```python
from build123d import *

# Parameters (mm, degrees)
BOSS_EXTRUDE1_DEPTH = 60
CUT_EXTRUDE1_DEPTH  = 10
CUT_EXTRUDE2_DEPTH  = 10
CUT_EXTRUDE3_DEPTH  = 30
SKETCH7_R           = 10
CUT_EXTRUDE5_DEPTH  = 75
SKETCH8_R           = 10
CUT_EXTRUDE6_DEPTH  = 75
SKETCH9_W           = 42
SKETCH9_H           = 40
CUT_EXTRUDE8_DEPTH  = 65
CUT_EXTRUDE9_DEPTH  = 10
CUT_EXTRUDE10_DEPTH = 20
SKETCH12_W          = 40
SKETCH12_H          = 10
CUT_EXTRUDE11_DEPTH = 20
BOSS_EXTRUDE2_DEPTH = 20
SKETCH14_R          = 10
CUT_EXTRUDE14_DEPTH = 20
CUT_EXTRUDE15_DEPTH = 10
BOSS_EXTRUDE3_DEPTH = 20
SKETCH18_R          = 10
CUT_EXTRUDE16_DEPTH = 20
CUT_EXTRUDE17_DEPTH = 10


with BuildPart() as part:
    # Sketch2 → Boss-Extrude1 (new body)
    with BuildSketch(Plane.XY):
        with BuildLine():
            Line((0, 0), (150, 0))
            Line((150, 0), (150, 70))
            Line((150, 70), (120, 70))
            Line((120, 70), (120, 40))
            Line((120, 40), (40, 40))
            ThreePointArc((40, 40), (11.715728753, 28.284271247), (0, 0))
        make_face()
    extrude(amount=BOSS_EXTRUDE1_DEPTH)

    # Sketch4 → Cut-Extrude1 (cut)
    with BuildSketch(Plane(origin=(150, 0, 0), x_dir=(0, 0, -1), z_dir=(1, 0, 0))):
        with BuildLine():
            Line((-50, 70), (-40, 70))
            ThreePointArc((-40, 70), (-30, 60), (-20, 70))
            Line((-20, 70), (-10, 70))
            ThreePointArc((-10, 70), (-30, 50), (-50, 70))
        make_face()
    extrude(amount=-CUT_EXTRUDE1_DEPTH, mode=Mode.SUBTRACT)

    # Sketch5 → Cut-Extrude2 (cut)
    with BuildSketch(Plane.ZY.offset(-120)):
        with BuildLine():
            Line((10, 70), (20, 70))
            ThreePointArc((20, 70), (30, 60), (40, 70))
            Line((40, 70), (50, 70))
            ThreePointArc((50, 70), (30, 50), (10, 70))
        make_face()
    extrude(amount=-CUT_EXTRUDE2_DEPTH, mode=Mode.SUBTRACT)

    # Sketch6 → Cut-Extrude3 (cut)
    with BuildSketch(Plane.ZY.offset(-120)):
        with BuildLine():
            Line((20, 70), (40, 70))
            ThreePointArc((40, 70), (30, 60), (20, 70))
        make_face()
    extrude(amount=-CUT_EXTRUDE3_DEPTH, mode=Mode.SUBTRACT)

    # Sketch7 → Cut-Extrude5 (cut)
    with BuildSketch(Plane(origin=(0, 40, 0), x_dir=(1, 0, 0), z_dir=(0, 1, 0))):
        with Locations((90, -30)):
            Circle(SKETCH7_R)
    extrude(amount=-CUT_EXTRUDE5_DEPTH, mode=Mode.SUBTRACT)

    # Sketch8 → Cut-Extrude6 (cut)
    with BuildSketch(Plane.XZ):
        with Locations((30, 30)):
            Circle(SKETCH8_R)
    extrude(amount=-CUT_EXTRUDE6_DEPTH, mode=Mode.SUBTRACT)

    # Sketch9 → Cut-Extrude8 (cut)
    with BuildSketch(Plane(origin=(0, 20, 0), x_dir=(1, 0, 0), z_dir=(0, 1, 0))):
        with Locations((29, -30)):
            Rectangle(SKETCH9_W, SKETCH9_H)
    extrude(amount=CUT_EXTRUDE8_DEPTH, mode=Mode.SUBTRACT)

    # Sketch10 → Cut-Extrude9 (cut)
    with BuildSketch(Plane(origin=(0, 40, 0), x_dir=(1, 0, 0), z_dir=(0, 1, 0))):
        with BuildLine():
            Line((90, -20), (50, -20))
            Line((50, -20), (50, -40))
            Line((50, -40), (90, -40))
            ThreePointArc((90, -40), (80, -30), (90, -20))
        make_face()
    extrude(amount=-CUT_EXTRUDE9_DEPTH, mode=Mode.SUBTRACT)

    # Sketch11 → Cut-Extrude10 (cut)
    with BuildSketch(Plane.XY.offset(20)):
        Polygon((50, 20), (70, 30), (50, 30), align=None)
    extrude(amount=CUT_EXTRUDE10_DEPTH, mode=Mode.SUBTRACT)

    # Sketch12 → Cut-Extrude11 (cut)
    with BuildSketch(Plane(origin=(0, 40, 0), x_dir=(1, 0, 0), z_dir=(0, 1, 0))):
        with Locations((90, -55)):
            Rectangle(SKETCH12_W, SKETCH12_H)
        with Locations((90, -5)):
            Rectangle(SKETCH12_W, SKETCH12_H)
    extrude(amount=-CUT_EXTRUDE11_DEPTH, mode=Mode.SUBTRACT)

    # Sketch13 → Boss-Extrude2 (add)
    with BuildSketch(Plane(origin=(0, 0, 0), x_dir=(1, 0, 0), z_dir=(0, 1, 0))):
        with BuildLine():
            Line((70, -70), (70, -80))
            ThreePointArc((70, -80), (90, -100), (110, -80))
            Line((110, -80), (110, -70))
            ThreePointArc((110, -70), (112.928932188, -62.928932188), (120, -60))
            Line((120, -60), (60, -60))
            ThreePointArc((60, -60), (67.071067812, -62.928932188), (70, -70))
        make_face()
    extrude(amount=BOSS_EXTRUDE2_DEPTH)

    # Sketch14 → Cut-Extrude14 (cut)
    with BuildSketch(Plane(origin=(0, 20, 0), x_dir=(1, 0, 0), z_dir=(0, 1, 0))):
        with Locations((90, -80)):
            Circle(SKETCH14_R)
    extrude(amount=-CUT_EXTRUDE14_DEPTH, mode=Mode.SUBTRACT)

    # Sketch15 → Cut-Extrude15 (cut)
    with BuildSketch(Plane(origin=(0, 20, 0), x_dir=(1, 0, 0), z_dir=(0, 1, 0))):
        with BuildLine():
            Line((70, -80), (80, -80))
            ThreePointArc((80, -80), (90, -90), (100, -80))
            Line((100, -80), (110, -80))
            ThreePointArc((110, -80), (90, -100), (70, -80))
        make_face()
    extrude(amount=-CUT_EXTRUDE15_DEPTH, mode=Mode.SUBTRACT)

    # Sketch17 → Boss-Extrude3 (add)
    with BuildSketch(Plane.XZ):
        with BuildLine():
            Line((110, -10), (110, -20))
            ThreePointArc((110, -20), (90, -40), (70, -20))
            Line((70, -20), (70, -10))
            ThreePointArc((70, -10), (67.071067812, -2.928932188), (60, 0))
            Line((60, 0), (120, 0))
            ThreePointArc((120, 0), (112.928932188, -2.928932188), (110, -10))
        make_face()
    extrude(amount=-BOSS_EXTRUDE3_DEPTH)

    # Sketch18 → Cut-Extrude16 (cut)
    with BuildSketch(Plane(origin=(0, 20, 0), x_dir=(1, 0, 0), z_dir=(0, 1, 0))):
        with Locations((90, 20)):
            Circle(SKETCH18_R)
    extrude(amount=-CUT_EXTRUDE16_DEPTH, mode=Mode.SUBTRACT)

    # Sketch19 → Cut-Extrude17 (cut)
    with BuildSketch(Plane(origin=(0, 20, 0), x_dir=(1, 0, 0), z_dir=(0, 1, 0))):
        with BuildLine():
            Line((100, 20), (110, 20))
            ThreePointArc((110, 20), (90, 40), (70, 20))
            Line((70, 20), (80, 20))
            ThreePointArc((80, 20), (90, 30), (100, 20))
        make_face()
    extrude(amount=-CUT_EXTRUDE17_DEPTH, mode=Mode.SUBTRACT)


solid = part.part
```
Source: CAD feature listing. Evaluate the final solid. Frame: model axes, mm. A direction names the side the tool comes from. Coordinates: 2 decimals unless noted, no trailing zeros. Loops run counter-clockwise (first coordinate to the right, second up) from the corner with the lowest first, then second, coordinate; pieces in that order, holes last. Notation, with made-up numbers: M 31,-12.5 L 71,-12.5 A5 ccw 71,-3.5 Z; hole C 59.25,81 d6. An arc over 180 degrees is marked long. Use a Markdown table: item, result. Add a question column.
Q1. Material intervals for L1, parallel to Z at x = 90, y = 9; L2, parallel to Z at x = 49, y = 36; L3, parallel to Z at x = 98, y = 6, sorted ascending.
Q2. Section query C-C, the plane y = 38. Return loops of the section in (x, z).
Q3. First-contact query: pin 1 (5 mm diameter, centred on x = 48, y = 13.5, fed in from +Z); pin 2 (12 mm diameter, centred on x = 30, z = 30, fed in from -Y); pin 3 (15 mm diameter, centred on y = 52.5, z = 28.5, fed in from -X); pin 4 (8 mm diameter, centred on x = 133, y = 18, fed in from -Z). Flat tips, straight axial feed; report the tip coordinate or a pass-through.
Q4. Section query D-D, the plane x = 30. Return loops of the section in (y, z).
Q5. Section query A-A, the plane z = 30. Return loops of the section in (x, y).
Q6. Section query B-B, the plane x = 82. Return loops of the section in (y, z).
Q7. Draft query along Z for faces 4 (the flat face through (50, 30, 15)), 5 (the cylindrical face through (90, 5, -40)), 6 (the flat face through (70, 10, -15)). Return one class per face: pulls with the +Z half, pulls with the -Z half, needs draft (parallel to the pull), parting line crosses it, or undercut.
Q8. Access query for faces 1 (the flat face through (75, 15, -20)), 2 (the flat face through (105, 15, 80)), 3 (the flat face through (70, 30, 55)). Directions: +Z, -Z, +X, -X, +Y, -Y. A direction counts if a zero-diameter tool reaches every point of the face in a straight line with its end or side. Return the directions, or none.
Result:
| question | item | result |
|---|---|---|
| 1 | L1 | z = -40 to -30, -10 to 20, 40 to 70, 90 to 100 |
| 1 | L2 | z = 0 to 10, 50 to 60 |
| 1 | L3 | z = -38.33 to -26, -14 to 24, 36 to 74, 86 to 98.33 |
| 2 | outline | M 27.51,0 L 70,0 L 70,10 L 110,10 L 110,0 L 150,0 L 150,60 L 110,60 L 110,50 L 70,50 L 70,60 L 27.51,60 L 27.51,50 L 50,50 L 50,40 L 90,40 A10 cw 90,20 L 50,20 L 50,10 L 27.51,10 Z |
| 3 | pin 1 | stops at z = 60 |
| 3 | pin 2 | passes through |
| 3 | pin 3 | stops at x = 120 |
| 3 | pin 4 | stops at z = 0 |
| 4 | outline | M 0,0 L 38.73,0 L 38.73,10 L 20,10 L 20,20 L 0,20 Z; M 0,40 L 20,40 L 20,50 L 38.73,50 L 38.73,60 L 0,60 Z |
| 5 | outline | M 0,0 L 20,0 L 20,20 L 8,20 L 8,24 A40 ccw Z; M 40,0 L 80,0 L 80,30 L 70,30 L 50,20 L 40,20 Z; M 100,0 L 150,0 L 150,50 L 140,50 L 140,60 L 130,60 L 130,50 L 120,50 L 120,40 L 100,40 Z |
| 6 | outline | M 0,-38.33 L 10,-38.33 L 10,-26 L 0,-26 Z; M 0,-14 L 20,-14 L 20,10 L 40,10 L 40,20 L 30,20 L 30,24 L 0,24 Z; M 0,36 L 30,36 L 30,40 L 40,40 L 40,50 L 20,50 L 20,74 L 0,74 Z; M 0,86 L 10,86 L 10,98.33 L 0,98.33 Z |
| 7 | face 4 | undercut |
| 7 | face 5 | pulls with the -Z half |
| 7 | face 6 | needs draft |
| 8 | face 1 | -Z, +X, -X, +Y |
| 8 | face 2 | +Z, +X, -X, +Y |
| 8 | face 3 | +Z, +Y |
